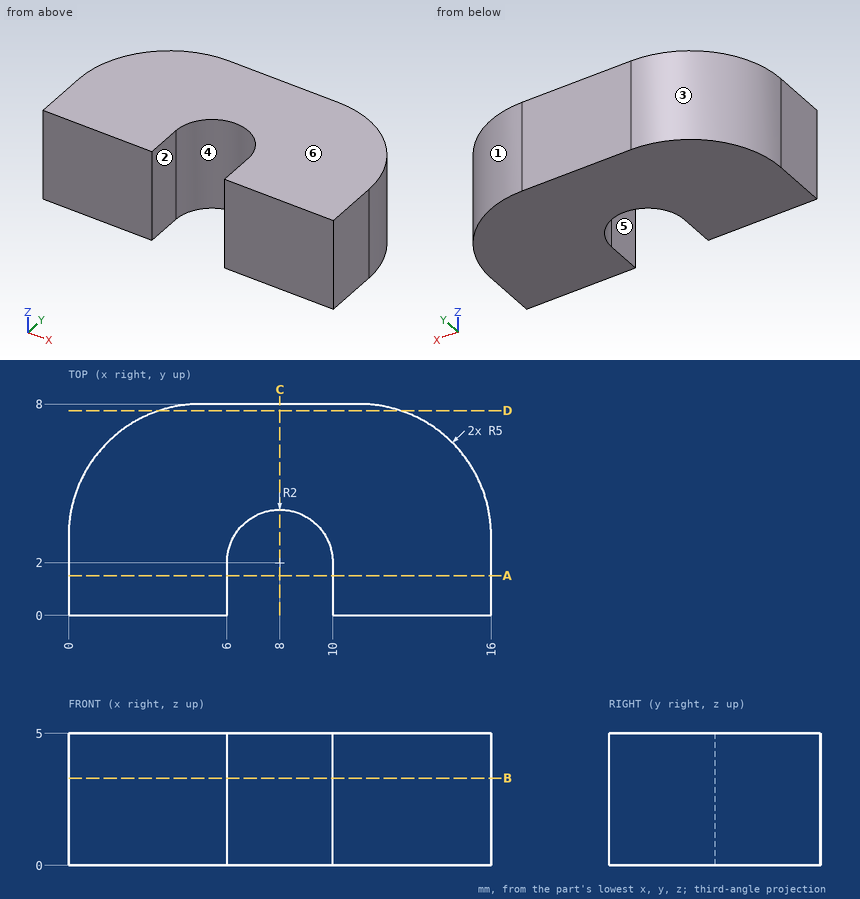
Input: dimensioned drawing with shaded views. Units: mm. Origin: part minimum x, y, z. A direction names the side the tool comes from. Give positions to 0.01 mm unless a question says otherwise; leave off trailing zeros. Loops run counter-clockwise (first coordinate to the right, second up) from the corner with the lowest first, then second, coordinate; pieces in that order, holes last. Notation, with made-up numbers: (-21, 23.5) -> (31, 23.5) arc R9 ccw to (31, 30.5) -> close; hole circle Ø3 at (6, 42.5). An arc over 180 degrees is marked (long way). Return JSON: item names as keys, results as strings.
Item 1: Section A-A, the plane y = 1.5. Output: boundary loops of the cut face in (x, z), plus the area to 3 significant figures.
Filled in:
{"outline": "(0, 0) -> (6, 0) -> (6, 5) -> (0, 5) -> close; (10, 0) -> (16, 0) -> (16, 5) -> (10, 5) -> close", "area": "60.0 mm^2"}
Item 2: Section D-D, the plane y = 7.75. Output: boundary loops of the cut face in (x, z).
Filled in:
{"outline": "(3.44, 0) -> (12.56, 0) -> (12.56, 5) -> (3.44, 5) -> close"}
Item 3: Access query for the marked faces 5 and 6. Directions: +Z, -Z, +X, -X, +Y, -Y. A direction counts if a zero-diameter tool reaches every point of the face in a straight line with its end or side. Return the directions, or none.
Filled in:
{"face 5": "+Z, -Z, -Y", "face 6": "+Z, +X, -X, +Y, -Y"}
Item 4: Pin query (flat end, axial travel): P1, Ø1.5, axis at y = 6.5, z = 4, coming from the +X side; P2, Ø2, axis at y = 4.5, z = 2, coming from the +X side; P3, Ø2, axis at y = 4.5, z = 2.5, coming from the -X side. Return the tip coordinate at first contact, or that it passes through.
Filled in:
{"P1": "x = 15.18", "P2": "x = 15.97", "P3": "x = 0.03"}
Item 5: Mould query, pull axis X, two halves, no side actions, for the marked faces 1, 2, 3 and 4. Classes: released by +X, released by -X, zero draft, split by the parting line, or undercut.
Filled in:
{"face 1": "released by +X", "face 2": "undercut", "face 3": "released by -X", "face 4": "undercut"}
Item 6: Line query: line 1 (X direction, y = 0.5, z = 2); line 2 (Y direction, x = 1, z = 2.1); line 3 (X direction, y = 2.5, z = 3.15). Output: solid intervals per line, ascending.
Filled in:
{"line 1": "0 to 6, 10 to 16", "line 2": "0 to 6", "line 3": "0 to 6.06, 9.94 to 16"}
Item 7: Section B-B, the plane z = 3.3. Output: boundary loops of the cut face in (x, y).
Filled in:
{"outline": "(0, 0) -> (6, 0) -> (6, 2) arc R2 cw to (10, 2) -> (10, 0) -> (16, 0) -> (16, 3) arc R5 ccw to (11, 8) -> (5, 8) arc R5 ccw to (0, 3) -> close"}
Item 8: Section C-C, the plane x = 8. Output: boundary loops of the cut face in (y, z), plus the area to 3 significant figures.
Filled in:
{"outline": "(4, 0) -> (8, 0) -> (8, 5) -> (4, 5) -> close", "area": "20.0 mm^2"}
